```python
from build123d import *

# Parameters (mm, degrees)
F3_DEPTH      = 50.8
F3_DEPTH_BACK = -50.8


with BuildPart() as f1:
    # F0 (on Front) → F1 (revolve)
    with BuildSketch(Plane.XZ):
        Polygon((-16.134506, -25.27852), (-6.990506, -25.27852), (-6.990506, 25.52148), (-16.134506, 25.52148), (-19.309506, 12.82148), (-19.309506, -12.57852), align=None)
    revolve(axis=Axis((-0.259506, 0, -0.29264), (0, 0, 1)))

    # F2 (on Top) → F3 (cut, two sides)
    with BuildSketch(Plane.XY) as f3_sk:
        Polygon((7.726794, 0.839726), (3.136173, 7.111463), (-4.590621, 6.271737), (-7.726794, -0.839726), (-3.136173, -7.111463), (4.590621, -6.271737), align=None)
    extrude(amount=-F3_DEPTH, mode=Mode.SUBTRACT)
    extrude(f3_sk.sketch, amount=-F3_DEPTH_BACK, mode=Mode.SUBTRACT)


solid = f1.part
```
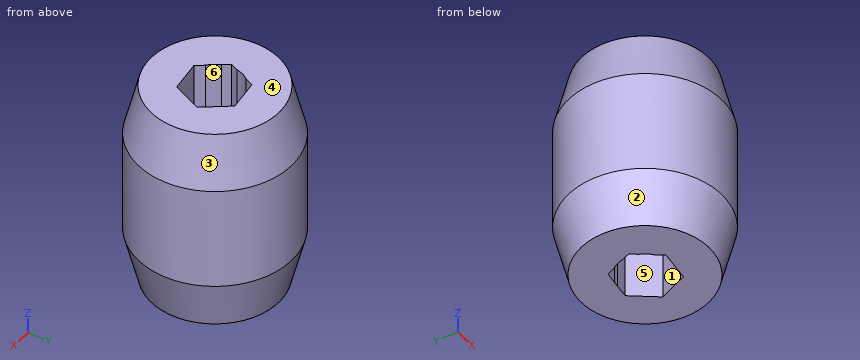
Part model, mm, in its own coordinate system. Face numbers are marked on the shaded views. A direction names the side the tool comes from. Give positions to 0.01 mm unless a question says otherwise; leave off trailing zeros. Order: outer loops, then holes, each group sorted by start corner. A loop starts at its lowest first (then second) coordinate and runs counter-clockwise, first axis right, second up. Notation, with made-up numbers: (85.25, 3.5) - (93.25, 3.5) arc R28 ccw to (93.25, 37.5) - close; hole circle Ø5 at (86, 39.5). An arc over 180 degrees is marked (long way). Use one line per item in the form item = value.
Item 1: Probe probe 1 along Y at (x, z) = (-3, 15.5); probe 2 along X at (y, z) = (-3, -16); probe 3 along Y at (x, z) = (-1, -5.5). List the from-to ranges inside material, lowest first. Write a range as from..to.
Solution:
probe_1 = -18.17..-7.1, 6.44..18.17
probe_2 = -18.21..-6.28, 6.03..17.69
probe_3 = -19.04..-6.88, 6.69..19.04
Item 2: Slice it at A-A on z = -2. Give the cut face in (x, y), and give its area (3 significant figures).
Solution:
outline = circle Ø38.1 at (-0.26, 0); hole (-7.73, -0.84) - (-6.51, -2.51) arc R6.73 ccw to (-4.54, -5.2) - (-3.14, -7.11) - (4.59, -6.27) - (7.73, 0.84) - (3.14, 7.11) - (-0.37, 6.73) arc R6.73 ccw to (-1.59, 6.6) - (-4.59, 6.27) - (-5.49, 4.24) arc R6.73 ccw to (-6.92, 1) - close
area = 982 mm2
Item 3: Slice it at B-B on y = 0. Give the cut face in (x, z), and give its area (3 significant figures).
Solution:
outline = (-19.31, -12.58) - (-16.13, -25.28) - (-7.36, -25.28) - (-7.36, 25.52) - (-16.13, 25.52) - (-19.31, 12.82) - close; (7.36, -25.28) - (15.62, -25.28) - (18.79, -12.58) - (18.79, 12.82) - (15.62, 25.52) - (7.36, 25.52) - close
area = 1,110 mm2
Item 4: Slice it at C-C on z = 16.5. Give the cut face in (x, y), and give its area (3 significant figures).
Solution:
outline = circle Ø36.26 at (-0.26, 0); hole (-7.73, -0.84) - (-6.51, -2.51) arc R6.73 ccw to (-4.54, -5.2) - (-3.14, -7.11) - (4.59, -6.27) - (7.73, 0.84) - (3.14, 7.11) - (-0.37, 6.73) arc R6.73 ccw to (-1.59, 6.6) - (-4.59, 6.27) - (-5.49, 4.24) arc R6.73 ccw to (-6.92, 1) - close
area = 875 mm2
Item 5: Pin check, flat tips, straight feed: pin 1 Ø10 at (x, y) = (-3.5, -1) entering from -Z; pin 2 Ø2 at (y, z) = (5, 7.5) entering from -X; pin 3 Ø6 at (x, z) = (-9.5, -6) entering from +Y; pin 4 Ø12 at (x, z) = (-1, -3) entering from -Y. Stop position of each tip, or through.
Solution:
pin_1 = -25.28
pin_2 = -18.88
pin_3 = 18
pin_4 = -19.05
Item 6: Two-plate mould, pull along Y, no slides. Class the marked faces 3, 4, 5 and 6: released by +Y, released by -Y, zero draft, split by the parting line, or undercut.
Solution:
face_3 = split by the parting line
face_4 = zero draft
face_5 = undercut
face_6 = undercut
Item 7: Which spindle directions (+Z, -Z, +X, -X, +Y, -Y) get a long thin tool onto all of the face, cutting with end or side? Do the marked faces 1 and 2. Say none if no direction does.
Solution:
face_1 = +Z, -Z
face_2 = -Z
